Model file for the job. Use its own axes, mm. A direction names the side the tool comes from. Round coordinates to 2 decimals unless told otherwise and drop trailing zeros. Loops run counter-clockwise (first coordinate to the right, second up) from the corner with the lowest first, then second, coordinate; pieces in that order, holes last. Notation, with made-up numbers: (15, -17.5) - (64, -17.5) arc R19 cw to (64, 14.5) - close; hole circle Ø2 at (45, 62.5). An arc over 180 degrees is marked (long way). Use one line per item in the form item = value.
Autodesk Inventor part; units mm, degrees
ref_plane "YZ Plane" through (0, 0, 0) normal (1, 0, 0) x (0, 1, 0)
ref_plane "XZ Plane" through (0, 0, 0) normal (0, 1, 0) x (-1, 0, 0)
ref_plane "XY Plane" through (0, 0, 0) normal (0, 0, 1) x (1, 0, 0)
sketch "arm_sketch" plane through (0, 0, 0) normal (0, 1, 0) x (-1, 0, 0)
  line L0 (0, -40) -> (-20, -40) construction
  line L1 (-20, -40) -> (-20, 0) construction
  line L2 (-20, 0) -> (0, 0) construction
  line L3 (0, 0) -> (0, -40) construction
  line L4 (0, -30) -> (-20, -30) construction
  line L5 (-20, -30) -> (-20, -10)
  line L6 (-20, -10) -> (0, -10) construction
  line L7 (0, -10) -> (0, -30) construction
  line L8 (-20, -40) -> (-34, -40)
  line L9 (-34, -40) -> (-34, -30)
  line L10 (-34, -30) -> (-20, -30)
  line L11 (-20, -30) -> (-20, -40) construction
  line L12 (0, -20) -> (-20, -20) construction
  line L13 (-10, -40) -> (-10, 0) construction
  line L14 (-20, 0) -> (-34, 0)
  line L15 (-34, 0) -> (-34, -10)
  line L16 (-34, -10) -> (-20, -10)
  line L17 (-20, -10) -> (-20, 0) construction
  line L18 (0, -40) -> (14, -40) construction
  line L19 (14, -40) -> (14, -30) construction
  line L20 (14, -30) -> (0, -30)
  line L21 (0, -30) -> (0, -40) construction
  line L22 (0, -10) -> (0, 0) construction
  line L23 (0, 0) -> (14, 0) construction
  line L24 (14, 0) -> (14, -10) construction
  line L25 (14, -10) -> (0, -10)
  line L26 (14, -30) -> (14, -10)
  line L27 (0, -10) -> (-8, -10)
  line L28 (-8, -10) -> (-8, 0)
  line L29 (0, -30) -> (-8, -30)
  line L30 (-8, -30) -> (-8, -40)
  line L31 (-8, -40) -> (-20, -40)
  line L32 (-8, 0) -> (-20, 0)
  point P0 (0, -10)
  point P1 (0, -10)
  dimension "d0" = 20
  dimension "d1" = 40
  dimension "d2" = 20
  dimension "d3" = 10
  dimension "d4" = 14
  dimension "d63" = 12
  dimension "d64" = 12
extrude "arm" add sketch "arm_sketch" along normal blind 10
sketch "Sketch5" plane through (8, 0, 0) normal (0, 0, 1) x (1, 0, 0)
  line L0 (26, 0) -> (26, 10) construction
  line L1 (26, 10) -> (12, 10) construction
  line L2 (-22, 0) -> (-22, 10) construction
  circle A0 centre (21, 5) radius 2
  circle A1 centre (-17, 5) radius 2
  dimension "d66" = 10
  dimension "d67" = 14
  dimension "d68" = 4
  dimension "d69" = 4
  dimension "d70" = 5
  dimension "d71" = 5
  dimension "d72" = 5
  dimension "d73" = 5
extrude "rod_hole" cut sketch "Sketch5" against normal through all
fillet "rot_round" radius 4 12 edges at (-14, 10, -20) (-14, 0, -20) (34, 10, -35) (34, 0, -35) (34, 10, -5) (34, 0, -5) (8, 10, -5) (8, 0, -5) (8, 0, -35) (8, 10, -35) (20, 10, -20) (20, 0, -20)
equation "\"d3\" = 0.5 * d1 - 0.5 * d2"
equation "\"d64\" = d63"
equation "\"d68\" = arm_rod_diam"
equation "\"d69\" = arm_rod_diam"
equation "\"d70\" = d71"
equation "\"d71\" = d72"
equation "\"d72\" = 0.5 * d66"
equation "\"d73\" = d72"
equation "\"d76\" = arm_rod_diam"
equation "\"arm_rod_diam\" = 4"
equation "\"hole\" = 2.2"
properties part number "arm" material "ABS Plastic"
1. Cut at A-A, the plane y = 5. Give the cut face in (x, z), plus the area to 3 significant figures.
Geometry check:
outline = (-14, -30) - (-11, -30) - (-11, -10) - (-14, -10) - close; (-7, -30) - (8, -30) - (8, -40) - (27, -40) - (27, -30) - (20, -30) - (20, -10) - (27, -10) - (27, 0) - (8, 0) - (8, -10) - (-7, -10) - close; (31, -40) - (34, -40) - (34, -30) - (31, -30) - close; (31, -10) - (34, -10) - (34, 0) - (31, 0) - close
area = 1,040 mm^2
2. Cut at B-B, the plane x = 29. Give the cut face in (y, z).
Geometry check:
outline = (0, -40) - (3, -40) - (3, -30) - (0, -30) - close; (0, -10) - (3, -10) - (3, 0) - (0, 0) - close; (7, -40) - (10, -40) - (10, -30) - (7, -30) - close; (7, -10) - (10, -10) - (10, 0) - (7, 0) - close
3. Wall check: probe 1 along Y at (x, z) = (29, -3.5); probe 2 along Z at (x, y) = (22.5, 2.25); probe 3 along X at (y, z) = (5.5, -15). Give the ranges that are in metal, low to high.
Geometry check:
probe_1 = 0 to 3, 7 to 10
probe_2 = -40 to -30, -10 to 0
probe_3 = -14 to -10.94, -7.06 to 20
4. Flat gauge pins, fed straight in: pin 1 (1.6 mm diameter, centred on y = 5, z = -21, fed in from +X); pin 2 (2.5 mm diameter, centred on x = 29, y = 5, fed in from +Z) (3 decimals); pin 3 (2 mm diameter, centred on y = 5, z = -36, fed in from -X); pin 4 (3 mm diameter, centred on x = -6.5, y = 5, fed in from -Z). Where does each tip first touch, or does it go through?
Geometry check:
pin_1 = 20
pin_2 = through
pin_3 = 8
pin_4 = -30
5. Cut at C-C, the plane x = -9. Give the cut face in (y, z).
Geometry check:
outline = (0, -30) - (3, -30) - (3, -10) - (0, -10) - close; (7, -30) - (10, -30) - (10, -10) - (7, -10) - close
6. Pull direction Z, two halves, no side cores. Call faces 6 (the flat face through (-1, 5, -30)), 7 (the cylindrical face through (18.797, 1.141, -19.86)), 8 (the cylindrical face through (32.797, 1.141, -34.93)): +Z half, -Z half, draft (parallel to the pull), parting line (faces both ways), or undercut.
Geometry check:
face_6 = -Z half
face_7 = undercut
face_8 = draft
7. Tool access for faces 1 (the cylindrical face through (9.203, 1.141, -35.07)), 2 (the flat face through (21, 5, -40)), 3 (the flat face through (10, 0, -20)), 4 (the cylindrical face through (9.141, 1.203, -4.93)), 5 (the cylindrical face through (18.859, 8.797, -19.86)): list every direction of +Z, -Z, +X, -X, +Y, -Y with a clear straight run to the whole face (end or side of a thin tool).
Geometry check:
face_1 = -Z, -X, -Y
face_2 = -Z, +X, -X, +Y, -Y
face_3 = +Z, -Z, +X, -X, -Y
face_4 = +Z, -X, -Y
face_5 = +X, +Y
8. Cut at D-D, the plane z = -20. Give the cut face in (x, y), plus the area to 3 significant figures.
Geometry check:
outline = (-14, 4) arc R4 ccw to (-10, 0) - (16, 0) arc R4 ccw to (20, 4) - (20, 6) arc R4 ccw to (16, 10) - (-10, 10) arc R4 ccw to (-14, 6) - close; hole circle Ø4 at (-9, 5)
area = 314 mm^2
